Study the drawing (mm; zero at the part's minimum x, y, z) and answer. A direction names the side the tool comes from. Give positions to 0.01 mm unless a question says otherwise; leave off trailing zeros. Order: outer loops, then holes, each group sorted by start corner. A loop starts at its lowest first (then second) coordinate and runs counter-clockwise, first axis right, second up.
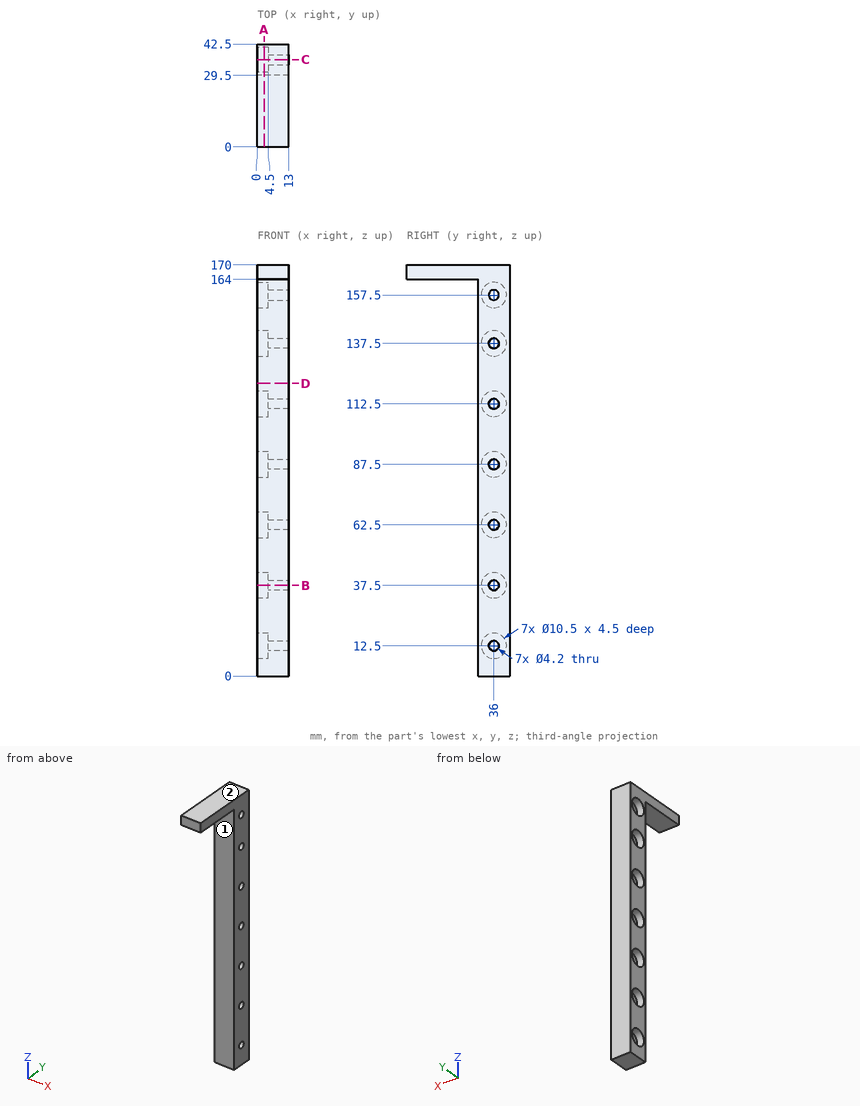
1) Find section B-B (z = 37.5). Write down the section's boundary in (x, y).
Geometry says:
outline: (0, 29.5) - (13, 29.5) - (13, 33.9) - (4.5, 33.9) - (4.5, 30.75) - (0, 30.75) - close; (0, 41.25) - (4.5, 41.25) - (4.5, 38.1) - (13, 38.1) - (13, 42.5) - (0, 42.5) - close
2) Straight lines are drawn through the part: probe 1 along Y at (x, z) = (8.75, 87.5); probe 2 along Y at (x, z) = (1.15, 12.5); probe 3 along Z at (x, y) = (1.5, 4). For each, find the intervals that lie inside material, in ascending order.
Geometry says:
probe 1: y = 29.5 to 33.9, 38.1 to 42.5
probe 2: y = 29.5 to 30.75, 41.25 to 42.5
probe 3: z = 164 to 170
3) A tool of negligible diameter and unlimited length cuts with its end or side. For the marked faces 1 and 2, from which of +Z, -Z, +X, -X, +Y, -Y can it reach the whole face along a straight path? Write none if from no direction.
Geometry says:
face 1: -Z, +X, -X, -Y
face 2: +Z, +X, -X, +Y, -Y
4) Find section D-D (z = 121). Write down the section's boundary in (x, y).
Geometry says:
outline: (0, 29.5) - (13, 29.5) - (13, 42.5) - (0, 42.5) - close
5) Find section A-A (x = 2.75). Write down the section's boundary in (y, z), then the cut area to 3 significant figures.
Geometry says:
outline: (0, 164) - (29.5, 164) - (29.5, 0) - (42.5, 0) - (42.5, 170) - (0, 170) - close; hole circle Ø10.5 at (36, 12.5); hole circle Ø10.5 at (36, 37.5); hole circle Ø10.5 at (36, 62.5); hole circle Ø10.5 at (36, 87.5); hole circle Ø10.5 at (36, 112.5); hole circle Ø10.5 at (36, 137.5); hole circle Ø10.5 at (36, 157.5)
area: 1,780 mm2
6) Find section C-C (y = 36). Count the separate pieces of the cut face and the enclosed holes in it, then the cut area to 3 significant figures.
Geometry says:
separate pieces: 8
enclosed holes: 0
area: 1,630 mm2
7) Given P1, Ø6.5, axis at x = 5, y = 22, coming from the -Z side; P2, Ø3, axis at y = 34.5, z = 65, coming from the -X side; P3, Ø4, axis at x = 9.5, z = 80, coming from the -Y side, each flat-ended and moving along its own axis, determine where each tip first touches the part or whether it passes through.
Geometry says:
P1: stops at z = 164
P2: stops at x = 4.5
P3: stops at y = 29.5
